```python
from build123d import *

# Parameters (mm, degrees)
SKETCH_1_R          = 14.5
EXTRUDE_1_DEPTH     = 1
SKETCH_3_R          = 8
EXTRUDE_3_DEPTH     = 21
SKETCH_4_W          = 2
SKETCH_4_H          = 13
CUT_EXTRUDE_1_DEPTH = 10
SKETCH_5_W          = 2
SKETCH_5_H          = 2
EXTRUDE_4_DEPTH     = 1


with BuildPart() as part:
    # 草图1 → 拉伸1 (new body)
    with BuildSketch(Plane(origin=(0, 0, 0), x_dir=(1, 0, 0), z_dir=(0, 1, 0))):
        with Locations(Location((0, 0, 0), (0, 0, 270))):
            Circle(SKETCH_1_R)
    extrude(amount=EXTRUDE_1_DEPTH)

    # 草图3 → 拉伸3 (add)
    with BuildSketch(Plane(origin=(0, 1, 0), x_dir=(-1, 0, 0), z_dir=(0, 1, 0))):
        with Locations(Location((0, 0, 0), (0, 0, 270))):
            Circle(SKETCH_3_R)
    extrude(amount=EXTRUDE_3_DEPTH)

    # 草图4 → 切除-拉伸1 (cut)
    with BuildSketch(Plane(origin=(0, 0, 0), x_dir=(-1, 0, 0), z_dir=(0, 1, 0))):
        Rectangle(SKETCH_4_W, SKETCH_4_H)
    extrude(amount=CUT_EXTRUDE_1_DEPTH, mode=Mode.SUBTRACT)

    # 草图5 → 拉伸4 (add)
    with BuildSketch(Plane.XZ.offset(-10)):
        Rectangle(SKETCH_5_W, SKETCH_5_H)
    extrude(amount=EXTRUDE_4_DEPTH)


solid = part.part
```
Input: part model. Units: mm. Frame: model coordinates. A direction names the side the tool comes from. Round coordinates to 2 decimals unless told otherwise and drop trailing zeros. Loops run counter-clockwise (first coordinate to the right, second up) from the corner with the lowest first, then second, coordinate; pieces in that order, holes last. Notation, with made-up numbers: M 46,-18 L 63,-18 A5 ccw 63,-13 Z; hole C -16,43 d2. An arc over 180 degrees is marked long. Answer in a Markdown table with one row per item. Add a question column.
1. Section B-B (z = 0). Output: boundary loops of the cut face in (x, y), and give its area (3 significant figures).
2. Section C-C (x = 0). Output: boundary loops of the cut face in (y, z), and give its area (3 significant figures).
3. Contact query for flat-ended pins moving along their axis: pin 1 (6 mm diameter, centred on y = 13, z = 10, fed in from +X); pin 2 (6 mm diameter, centred on x = 9.5, y = 14, fed in from +Z); pin 3 (3 mm diameter, centred on x = 2, z = 9, fed in from -Y); pin 4 (8 mm diameter, centred on x = -4.5, y = 8, fed in from -Z). Output: stop coordinate, or through.
4. Set-up query: faces 1 (the face through (7.81, 11.35, 1.73)), 2 (the face through (0, 10, 4)), 3 (the face through (-3, 0, 0)). Return all of +Z, -Z, +X, -X, +Y, -Y with unobstructed straight access to the full face (end or side cutting, diameter ignored); none if empty.
5. Section D-D (y = 1.75). Output: boundary loops of the cut face in (x, z).
6. Mould query, pull axis Z, two halves, no side actions, for faces 4 (the face through (-5.554, 0.493, 13.394)), 5 (the face through (-6, 1, 6)), 6 (the face through (1, 5, 0)). Classes: released by +Z, released by -Z, zero draft, split by the parting line, or undercut.
7. Section A-A (y = 9.5). Output: boundary loops of the cut face in (x, z).
8. Ray query, probe 1 along Y at (x, z) = (-13, 4.25); probe 2 along X at (y, z) = (4.5, 5.5); probe 3 along X at (y, z) = (15.25, 0). Return the intervals inside material, ascending.
Values follow:
| question | item | result |
|---|---|---|
| 1 | outline | M -14.5,0 L -1,0 L -1,9 L 1,9 L 1,0 L 14.5,0 L 14.5,1 L 8,1 L 8,22 L -8,22 L -8,1 L -14.5,1 Z |
| 1 | area | 347 mm^2 |
| 2 | outline | M 0,-14.5 L 1,-14.5 L 1,-8 L 22,-8 L 22,8 L 1,8 L 1,14.5 L 0,14.5 L 0,6.5 L 10,6.5 L 10,1 L 9,1 L 9,-1 L 10,-1 L 10,-6.5 L 0,-6.5 Z |
| 2 | area | 237 mm^2 |
| 3 | pin 1 | x = 3.87 |
| 3 | pin 2 | z = 4.66 |
| 3 | pin 3 | y = 0 |
| 3 | pin 4 | z = -7.98 |
| 4 | face 1 | +Y |
| 4 | face 2 | -Y |
| 4 | face 3 | +Z, -Z, +X, -X, -Y |
| 5 | outline | C 0,0 d16; hole M -1,-6.5 L 1,-6.5 L 1,6.5 L -1,6.5 Z |
| 6 | face 4 | split by the parting line |
| 6 | face 5 | zero draft |
| 6 | face 6 | undercut |
| 7 | outline | C 0,0 d16; hole M -1,-6.5 L 1,-6.5 L 1,-1 L -1,-1 Z; hole M -1,1 L 1,1 L 1,6.5 L -1,6.5 Z |
| 8 | probe 1 | 0 to 1 |
| 8 | probe 2 | -5.81 to -1, 1 to 5.81 |
| 8 | probe 3 | -8 to 8 |
